Verification items for the finished model (mm, model axes). Face numbers are marked on the shaded views. A direction names the side the tool comes from. Round coordinates to 2 decimals unless told otherwise and drop trailing zeros. Loops run counter-clockwise (first coordinate to the right, second up) from the corner with the lowest first, then second, coordinate; pieces in that order, holes last.
from build123d import *

# Parameters (mm, degrees)
SKETCH1_W                      = 134
SKETCH1_H                      = 74
SKETCH1_W_2                    = 62
SKETCH1_H_2                    = 40
BOSS_EXTRUDE1_DEPTH            = 120
CUT_EXTRUDE1_DEPTH             = 30
SKETCH4_W                      = 32
SKETCH4_H                      = 58
CUT_EXTRUDE2_DEPTH             = 42
SKETCH5_W                      = 32
SKETCH5_H                      = 116
CUT_EXTRUDE3_DEPTH             = 42
M2_5_CLEARANCE_HOLE1_D         = 2.9
M2_5_CLEARANCE_HOLE1_DEPTH     = 14
M2_5_CLEARANCE_HOLE1_TIP       = 0.386628252
SKETCH9_W                      = 40
SKETCH9_H                      = 56
CUT_EXTRUDE9_DEPTH             = 32
CUT_EXTRUDE5_DEPTH             = 20
CUT_EXTRUDE6_DEPTH             = 10
SKETCH12_W                     = 5
SKETCH12_H                     = 10
BOSS_EXTRUDE2_DEPTH            = 10
SKETCH13_R                     = 2.5
BOSS_EXTRUDE4_DEPTH            = 15
SKETCH14_W                     = 5
SKETCH14_H                     = 10
BOSS_EXTRUDE3_DEPTH            = 19.99
SKETCH17_W                     = 10
SKETCH17_H                     = 10
CUT_EXTRUDE10_DEPTH            = 5
SKETCH18_R                     = 2.5
BOSS_EXTRUDE5_DEPTH            = 15
CUT_EXTRUDE11_START            = -5
SKETCH19_R                     = 2.5
SKETCH19_R_2                   = 0.75
CUT_EXTRUDE11_DEPTH            = 5
SKETCH24_W                     = 5.919805253
SKETCH24_H                     = 2
BOSS_EXTRUDE6_DEPTH            = 10
CUT_EXTRUDE14_REACH            = 146.395
SKETCH26_W                     = 10
SKETCH26_H                     = 2.941902197
BOSS_EXTRUDE7_DEPTH            = 10
CUT_EXTRUDE15_REACH            = 146.819
SKETCH30_W                     = 3.947736589
SKETCH30_H                     = 10
BOSS_EXTRUDE8_DEPTH            = 10
CUT_EXTRUDE18_REACH            = 176.552
SKETCH33_W                     = 42
SKETCH33_H                     = 58
SKETCH33_W_2                   = 40
SKETCH33_H_2                   = 56
CUT_EXTRUDE20_DEPTH            = 2
CUT_EXTRUDE21_REACH            = 151.943
SKETCH34_R                     = 2
SKETCH36_W                     = 3
SKETCH36_H                     = 4
SUPORTE_DA_TAMPA_PILHA_DEPTH   = 5
SKETCH37_W                     = 3
SKETCH37_H                     = 3
SUPORTE_DA_TAMPA_2_PILHA_DEPTH = 4


with BuildPart() as part:
    # Sketch1 → Boss-Extrude1 (new body)
    with BuildSketch(Plane(origin=(0, 0, 0), x_dir=(1, 0, 0), z_dir=(0, 1, 0))):
        with Locations((11.401433692, -11.808243728)):
            Rectangle(SKETCH1_W, SKETCH1_H)
        with Locations((11.401433692, -26.808243728)):
            Rectangle(SKETCH1_W_2, SKETCH1_H_2, mode=Mode.SUBTRACT)
    extrude(amount=-BOSS_EXTRUDE1_DEPTH)

    # Sketch2 → Cut-Extrude1 (cut)
    with BuildSketch(Plane(origin=(0, 0, -25.191756272), x_dir=(-1, 0, 0), z_dir=(0, 0, -1))):
        Polygon((21.598566308, -118), (-64.401433692, -118), (-64.401433692, -106), (-76.401433692, -106), (-76.401433692, -14), (-64.401433692, -14), (-64.401433692, -2), (41.598566308, -2), (41.598566308, -14), (53.598566308, -14), (53.598566308, -88), (21.598566308, -88), align=None)
    extrude(amount=-CUT_EXTRUDE1_DEPTH, mode=Mode.SUBTRACT)

    # Sketch4 → Cut-Extrude2 (cut)
    with BuildSketch(Plane(origin=(0, 0, 4.808243728), x_dir=(-1, 0, 0), z_dir=(0, 0, -1))):
        with Locations((37.598566308, -31)):
            Rectangle(SKETCH4_W, SKETCH4_H)
    extrude(amount=-CUT_EXTRUDE2_DEPTH, mode=Mode.SUBTRACT)

    # Sketch5 → Cut-Extrude3 (cut)
    with BuildSketch(Plane(origin=(0, 0, 4.808243728), x_dir=(-1, 0, 0), z_dir=(0, 0, -1))):
        with Locations((-60.401433692, -60)):
            Rectangle(SKETCH5_W, SKETCH5_H)
    extrude(amount=-CUT_EXTRUDE3_DEPTH, mode=Mode.SUBTRACT)

    # M2.5 Clearance Hole1
    with Locations(Plane(origin=(0, 0, -25.191756272), x_dir=(-1, 0, 0), z_dir=(0, 0, -1))):
        with Locations((-70.401433692, -8), (47.598566308, -8), (47.598566308, -112), (-70.401433692, -112)):
            Hole(M2_5_CLEARANCE_HOLE1_D / 2, depth=M2_5_CLEARANCE_HOLE1_DEPTH)
            with Locations((0, 0, -(M2_5_CLEARANCE_HOLE1_DEPTH + M2_5_CLEARANCE_HOLE1_TIP / 2))):  # 150.14° drill point
                Cone(0, M2_5_CLEARANCE_HOLE1_D / 2, M2_5_CLEARANCE_HOLE1_TIP, mode=Mode.SUBTRACT)

    # Sketch9 → Cut-Extrude9 (cut)
    with BuildSketch(Plane.ZY.offset(55.598566308)):
        with Locations((26.808243728, -90)):
            Rectangle(SKETCH9_W, SKETCH9_H)
    extrude(amount=-CUT_EXTRUDE9_DEPTH, mode=Mode.SUBTRACT)

    # Sketch10 → Cut-Extrude5 (cut)
    with BuildSketch(Plane(origin=(0, 0, -25.191756272), x_dir=(-1, 0, 0), z_dir=(0, 0, -1))):
        Polygon((21.598566308, -88), (53.598566308, -88), (53.598566308, -106), (41.598566308, -106), (41.598566308, -118), (21.598566308, -118), align=None)
    extrude(amount=-CUT_EXTRUDE5_DEPTH, mode=Mode.SUBTRACT)

    # Sketch11 → Cut-Extrude6 (cut)
    with BuildSketch(Plane(origin=(0, 0, -5.191756272), x_dir=(-1, 0, 0), z_dir=(0, 0, -1))):
        Polygon((53.598566308, -88), (21.598566308, -88), (21.598566308, -118), (41.598566308, -118), (41.598566308, -106), (53.598566308, -106), align=None)
    extrude(amount=-CUT_EXTRUDE6_DEPTH, mode=Mode.SUBTRACT)

    # Sketch12 → Boss-Extrude2 (add)
    with BuildSketch(Plane(origin=(44.401433692, 0, 0), x_dir=(0, 0, -1), z_dir=(1, 0, 0))):
        with Locations((-7.308243728, -7)):
            Rectangle(SKETCH12_W, SKETCH12_H)
        with Locations((-7.308243728, -113)):
            Rectangle(SKETCH12_W, SKETCH12_H)
    extrude(amount=BOSS_EXTRUDE2_DEPTH)

    # Sketch13 → Boss-Extrude4 (add)
    with BuildSketch(Plane(origin=(0, 0, 4.808243728), x_dir=(-1, 0, 0), z_dir=(0, 0, -1))):
        with Locations(Location((-49.401433692, -7, 0), (0, 0, 180))):
            Circle(SKETCH13_R)
        with Locations(Location((-49.401433692, -113, 0), (0, 0, 180))):
            Circle(SKETCH13_R)
    extrude(amount=BOSS_EXTRUDE4_DEPTH)

    # Sketch14 → Boss-Extrude3 (add)
    with BuildSketch(Plane.ZY.offset(21.598566308)):
        with Locations((7.308243728, -7)):
            Rectangle(SKETCH14_W, SKETCH14_H)
    extrude(amount=BOSS_EXTRUDE3_DEPTH)

    # Sketch17 → Cut-Extrude10 (cut)
    with BuildSketch(Plane(origin=(0, 0, 4.808243728), x_dir=(-1, 0, 0), z_dir=(0, 0, -1))):
        with Locations((26.598566308, -7)):
            Rectangle(SKETCH17_W, SKETCH17_H)
    extrude(amount=-CUT_EXTRUDE10_DEPTH, mode=Mode.SUBTRACT)

    # Sketch18 → Boss-Extrude5 (add)
    with BuildSketch(Plane(origin=(0, 0, 4.808243728), x_dir=(-1, 0, 0), z_dir=(0, 0, -1))):
        with Locations((36.598571318, -7)):
            Circle(SKETCH18_R)
        with Locations((37.337526325, -113.738960016)):
            Circle(SKETCH18_R)
    extrude(amount=BOSS_EXTRUDE5_DEPTH)

    # Sketch19 → Cut-Extrude11 (cut)
    # profile 1 of 4: a face of its own
    with BuildSketch(Plane(origin=(0, 0, -10.191756272), x_dir=(-1, 0, 0), z_dir=(0, 0, -1)).offset(CUT_EXTRUDE11_START)):
        with Locations(Location((-49.401433692, -113, 0), (0, 0, 180))):
            Circle(SKETCH19_R)
        with Locations((-49.401433692, -113)):
            Circle(SKETCH19_R_2, mode=Mode.SUBTRACT)
    # profile 2 of 4: a face of its own
    with BuildSketch(Plane(origin=(0, 0, -10.191756272), x_dir=(-1, 0, 0), z_dir=(0, 0, -1)).offset(CUT_EXTRUDE11_START)):
        with Locations(Location((-49.401433692, -7, 0), (0, 0, 180))):
            Circle(SKETCH19_R)
        with Locations((-49.401433692, -7)):
            Circle(SKETCH19_R_2, mode=Mode.SUBTRACT)
    # profile 3 of 4: a face of its own
    with BuildSketch(Plane(origin=(0, 0, -10.191756272), x_dir=(-1, 0, 0), z_dir=(0, 0, -1)).offset(CUT_EXTRUDE11_START)):
        with Locations((36.598571318, -7)):
            Circle(SKETCH19_R)
        with Locations((36.598571318, -7)):
            Circle(SKETCH19_R_2, mode=Mode.SUBTRACT)
    # profile 4 of 4: a face of its own
    with BuildSketch(Plane(origin=(0, 0, -10.191756272), x_dir=(-1, 0, 0), z_dir=(0, 0, -1)).offset(CUT_EXTRUDE11_START)):
        with Locations((37.337526325, -113.738960016)):
            Circle(SKETCH19_R)
        with Locations((37.337526325, -113.738960016)):
            Circle(SKETCH19_R_2, mode=Mode.SUBTRACT)
    extrude(amount=CUT_EXTRUDE11_DEPTH, mode=Mode.SUBTRACT)

    # Sketch24 → Boss-Extrude6 (add)
    with BuildSketch(Plane.XY.offset(9.808243728)):
        with Locations((47.361336319, -8)):
            Rectangle(SKETCH24_W, SKETCH24_H)
    extrude(amount=BOSS_EXTRUDE6_DEPTH)

    # Sketch25 → Cut-Extrude14 (cut, up to next)
    with BuildSketch(Plane.XZ.offset(9), mode=Mode.PRIVATE) as cut_extrude14_sk1:
        Polygon((50.321238945, 9.808243728), (44.401433692, 19.808243728), (50.321238945, 19.808243728), align=None)
    cut_extrude14_tool1 = extrude(cut_extrude14_sk1.sketch, amount=-CUT_EXTRUDE14_REACH, mode=Mode.PRIVATE) & part.part
    add(cut_extrude14_tool1.solids().sort_by_distance((48.347971, -9, 16.47491))[0], mode=Mode.SUBTRACT)

    # Sketch26 → Boss-Extrude7 (add)
    with BuildSketch(Plane.XY.offset(9.808243728)):
        with Locations((49.401433692, -113.021848151)):
            Rectangle(SKETCH26_W, SKETCH26_H)
    extrude(amount=BOSS_EXTRUDE7_DEPTH)

    # Sketch27 → Cut-Extrude15 (cut, up to next)
    with BuildSketch(Plane(origin=(0, -111.550897052, 0), x_dir=(1, 0, 0), z_dir=(0, 1, 0)), mode=Mode.PRIVATE) as cut_extrude15_sk1:
        Polygon((54.401433692, -9.808243728), (44.401433692, -19.808243728), (54.401433692, -19.808243728), align=None)
    cut_extrude15_tool1 = extrude(cut_extrude15_sk1.sketch, amount=-CUT_EXTRUDE15_REACH, mode=Mode.PRIVATE) & part.part
    add(cut_extrude15_tool1.solids().sort_by_distance((51.0681, -111.550897, 16.47491))[0], mode=Mode.SUBTRACT)

    # Sketch30 → Boss-Extrude8 (add)
    with BuildSketch(Plane.XY.offset(9.808243728)):
        with Locations((-36.612321656, -7)):
            Rectangle(SKETCH30_W, SKETCH30_H)
    extrude(amount=BOSS_EXTRUDE8_DEPTH)

    # Sketch31 → Cut-Extrude18 (cut, up to next)
    with BuildSketch(Plane.ZY.offset(38.58618995), mode=Mode.PRIVATE) as cut_extrude18_sk1:
        Polygon((19.808243728, -2), (19.808243728, -12), (9.808243728, -12), align=None)
    cut_extrude18_tool1 = extrude(cut_extrude18_sk1.sketch, amount=-CUT_EXTRUDE18_REACH, mode=Mode.PRIVATE) & part.part
    add(cut_extrude18_tool1.solids().sort_by_distance((-38.58619, -8.666667, 16.47491))[0], mode=Mode.SUBTRACT)

    # Sketch33 → Cut-Extrude20 (cut)
    with BuildSketch(Plane.ZY.offset(55.598566308)):
        with Locations((26.808243728, -90)):
            Rectangle(SKETCH33_W, SKETCH33_H)
        with Locations((26.808243728, -90)):
            Rectangle(SKETCH33_W_2, SKETCH33_H_2, mode=Mode.SUBTRACT)
    extrude(amount=-CUT_EXTRUDE20_DEPTH, mode=Mode.SUBTRACT)

    # Sketch34 → Cut-Extrude21 (cut, up to next)
    with BuildSketch(Plane(origin=(0, 0, 4.808243728), x_dir=(-1, 0, 0), z_dir=(0, 0, -1)), mode=Mode.PRIVATE) as cut_extrude21_sk1:
        with Locations((37.530823831, -66.434778505)):
            Circle(SKETCH34_R)
    cut_extrude21_tool1 = extrude(cut_extrude21_sk1.sketch, amount=-CUT_EXTRUDE21_REACH, mode=Mode.PRIVATE) & part.part
    add(cut_extrude21_tool1.solids().sort_by_distance((-37.530824, -66.434779, 4.808244))[0], mode=Mode.SUBTRACT)

    # Sketch36 → Suporte da Tampa - Pilha (add)
    with BuildSketch(Plane(origin=(0, 0, 46.808243728), x_dir=(-1, 0, 0), z_dir=(0, 0, -1))):
        with Locations((49.098566308, -116)):
            Rectangle(SKETCH36_W, SKETCH36_H)
        with Locations((49.098566308, -64)):
            Rectangle(SKETCH36_W, SKETCH36_H)
    extrude(amount=SUPORTE_DA_TAMPA_PILHA_DEPTH)

    # Sketch37 → Suporte da Tampa 2 - Pilha (add)
    with BuildSketch(Plane.XY.offset(6.808243728)):
        with Locations((-49.098566308, -116.5)):
            Rectangle(SKETCH37_W, SKETCH37_H)
        with Locations((-49.098566308, -63.5)):
            Rectangle(SKETCH37_W, SKETCH37_H)
    extrude(amount=SUPORTE_DA_TAMPA_2_PILHA_DEPTH)


solid = part.part
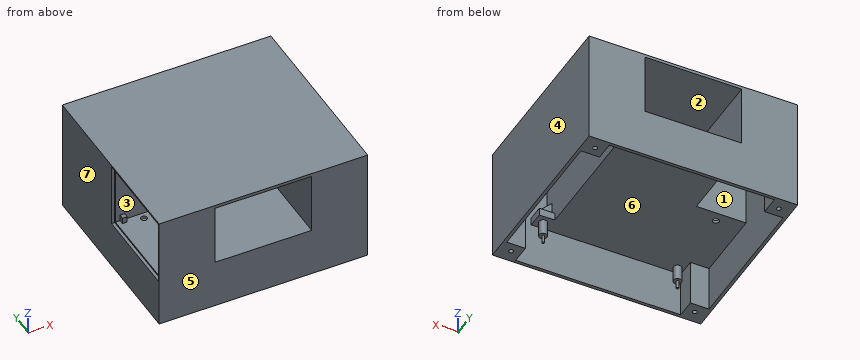
1. Section check B-B (x = -5.5). Enter the section's corners in (y, z).
2. Section check A-A (z = 39). Enter the section's corners in (x, y), then the cut area to 3 significant figures.
3. Section check D-D (x = -30). Enter the section's corners in (y, z).
4. Release check for a two-part mould opening along Y. For the marked faces 5, 6 and 7 record: released by +Y, released by -Y, zero draft, split by the parting line, or undercut.
5. Scan lines: L1, parallel to X at y = -93, z = 45; L2, parallel to X at y = -112, z = -14; L3, parallel to Y at x = -46.5, z = 12. Record each from-to range of solid material in increasing order.
6. Tool access check on the marked faces 1, 2, 3 and 4. Record the directions out of +Z, -Z, +X, -X, +Y, -Y that give a thin tool (end or side, any length) a straight path to the whole face; none if there is none.
7. Section check C-C (y = -46.5). Enter the section's corners in (x, z).
8. Gauge pin test, flat ends, axial feed: P1, Ø8, axis at x = 38, y = -55, coming from the -Z side; P2, Ø3, axis at y = -115.5, z = 44.5, coming from the -X side. Record the tip position at first contact, or that the pin passes through.
Taken from the geometry:
1. outline: (-120, -25.19) - (-118, -25.19) - (-118, 4.81) - (-2, 4.81) - (-2, -25.19) - (0, -25.19) - (0, 6.81) - (-120, 6.81) - close; (-120, 46.81) - (0, 46.81) - (0, 48.81) - (-120, 48.81) - close
2. outline: (-55.6, -120) - (-19.6, -120) - (-19.6, 0) - (-55.6, 0) - (-55.6, -61) - (-53.6, -61) - (-53.6, -62) - (-23.6, -62) - (-23.6, -118) - (-53.6, -118) - (-53.6, -119) - (-55.6, -119) - close; (42.4, -120) - (78.4, -120) - (78.4, 0) - (42.4, 0) - close; hole (-53.6, -60) - (-21.6, -60) - (-21.6, -2) - (-53.6, -2) - close; hole (44.4, -118) - (76.4, -118) - (76.4, -2) - (44.4, -2) - close
2. area: 1,280 mm2
3. outline: (-120, -25.19) - (-118, -25.19) - (-118, 4.81) - (-60, 4.81) - (-60, 46.81) - (-2, 46.81) - (-2, -25.19) - (0, -25.19) - (0, 48.81) - (-120, 48.81) - close; hole (-118, 6.81) - (-62, 6.81) - (-62, 46.81) - (-118, 46.81) - close
4. face 5: released by -Y
4. face 6: undercut
4. face 7: zero draft
5. L1: x = -23.6 to -19.6, 42.4 to 44.4, 76.4 to 78.4
5. L2: x = -55.6 to -49.05, -46.15 to -41.6, 64.4 to 68.95, 71.85 to 78.4
5. L3: y = -120 to -118, -62 to -60, -2 to 0
6. face 1: -Z
6. face 2: +Y, -Y
6. face 3: none
6. face 4: +Z, -Z, +X, +Y, -Y
7. outline: (-55.6, -25.19) - (-53.6, -25.19) - (-53.6, 46.81) - (-21.6, 46.81) - (-21.6, 4.81) - (44.4, 4.81) - (44.4, 46.81) - (76.4, 46.81) - (76.4, -25.19) - (78.4, -25.19) - (78.4, 48.81) - (-55.6, 48.81) - close; hole (-19.6, 6.81) - (42.4, 6.81) - (42.4, 46.81) - (-19.6, 46.81) - close
8. P1: stops at z = 4.81
8. P2: stops at x = -50.6
